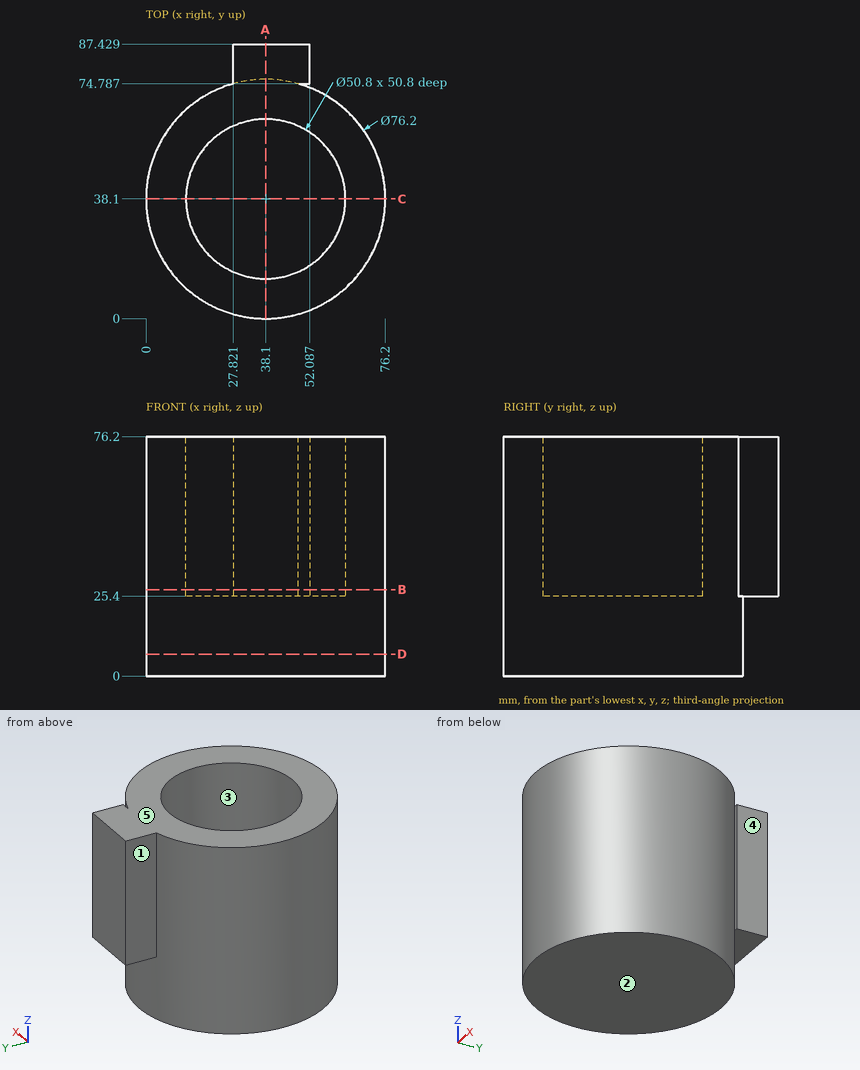
Source: three-view drawing plus pictorial views. Frame: mm from the lowest corner of the part. A direction names the side the tool comes from. Give positions to 0.01 mm unless a question says otherwise; leave off trailing zeros. Write each loop counter-clockwise with the first axis right and the second up, starting at its lowest first coordinate (ties: lowest second). Pieces come first, ordered by that corner, then holes. Notation, with made-up numbers: (11.5, 5.5) - (21.5, 5.5) arc R19 ccw to (21.5, 31.5) - close; hole circle Ø9 at (2.5, -27.5). An arc over 180 degrees is marked (long way). Write item = value, one per line. Start each with the question number.
Q1. Cut plane C-C, the plane y = 38.1. Return loops of the section in (x, z), then the cut area to 3 significant figures.
Q2. Draft query along X for the marked faces 3, 4 and 5. Return one class per face: +X half, -X half, draft (parallel to the pull), parting line (faces both ways), or undercut.
Q3. Cut plane A-A, the plane x = 38.1. Return loops of the section in (y, z).
Q4. Cut plane B-B, the plane z = 27.5. Return loops of the section in (x, y), then the cut area to 3 significant figures.
Q5. Material intervals for probe 1 along Y at (x, z) = (38, 63); probe 2 along X at (y, z) = (38, 36); probe 3 along Y at (x, z) = (50, 64) (1 decimal), sorted ascending.
Q6. Pin query (flat end, axial travel): pin 1 Ø4 at (y, z) = (83, 43) entering from -X; pin 2 Ø2 at (x, z) = (42, 12.5) entering from -Y; pin 3 Ø2 at (x, z) = (37.5, 53) entering from -Y. Return the tip coordinate at first contact, or that it passes through.
Q7. Cut plane D-D, the plane z = 7. Return loops of the section in (x, y).
Q8. Reachability of the marked faces 1 and 2 from +Z, -Z, +X, -X, +Y, -Y: full face, straight path, thin tool, end or side. Return the list, or none.
Computed values:
q1.outline = (0, 0) - (76.2, 0) - (76.2, 76.2) - (63.5, 76.2) - (63.5, 25.4) - (12.7, 25.4) - (12.7, 76.2) - (0, 76.2) - close
q1.area = 3,230 mm²
q2.face_3 = undercut
q2.face_4 = +X half
q2.face_5 = draft
q3.outline = (0, 0) - (76.2, 0) - (76.2, 25.4) - (87.43, 25.4) - (87.43, 76.2) - (63.5, 76.2) - (63.5, 25.4) - (12.7, 25.4) - (12.7, 76.2) - (0, 76.2) - close
q4.outline = (27.82, 74.79) arc R38.1 ccw (long way) to (48.38, 74.79) - (52.09, 74.79) - (52.09, 87.43) - (27.82, 87.43) - close; hole circle Ø50.8 at (38.1, 38.1)
q4.area = 2,820 mm²
q5.probe_1 = 0 to 12.7, 63.5 to 87.43
q5.probe_2 = 0 to 12.7, 63.5 to 76.2
q5.probe_3 = 1.9 to 15.7, 60.5 to 74.3, 74.8 to 87.4
q6.pin_1 = 27.82
q6.pin_2 = 0.11
q6.pin_3 = 0
q7.outline = circle Ø76.2 at (38.1, 38.1)
q8.face_1 = +Z, -Z, -X, +Y
q8.face_2 = -Z, +X, -X, +Y, -Y
